Could you check a few things on this model? Use its own coordinates, in mm. Face numbers are marked on the shaded views. A direction names the side the tool comes from. Give positions to 0.01 mm unless a question says otherwise; leave off trailing zeros. Loops run counter-clockwise (first coordinate to the right, second up) from the corner with the lowest first, then second, coordinate; pieces in that order, holes last. Notation, with made-up numbers: (-15.75, 23.5) - (-9.75, 23.5) arc R24 cw to (-9.75, 48.5) - close; hole circle Ø4 at (46, 63). An arc over 180 degrees is marked (long way). Write each question's results on one line, items separated by ' | '. Start each with the question number.
```python
from build123d import *
from build123d.topology import SkipClean

# Parameters (mm, degrees)
SKETCH_1_R          = 1.000029699
SKETCH_1_R_2        = 1.000000092
EXTRUDE_1_DEPTH     = 5
SKETCH_2_W          = 21.526040124
SKETCH_2_H          = 12.5
EXTRUDE_2_DEPTH     = 1.68
SKETCH_3_R          = 0.95
CUT_EXTRUDE_1_DEPTH = 5
SKETCH_4_W          = 12
SKETCH_4_H          = 4.5
SKETCH_4_R          = 1.000000092
EXTRUDE_3_DEPTH     = 7.05
SKETCH_5_R          = 1.149999977
EXTRUDE_4_DEPTH     = 6
CUT_EXTRUDE_START   = -5
SKETCH_6_R          = 0.95
CUT_EXTRUDE_2_DEPTH = 5
SKETCH_7_R          = 1
CUT_EXTRUDE_3_DEPTH = 100
SKETCH_8_R          = 1
CUT_EXTRUDE_4_DEPTH = 3
CUT_EXTRUDE_START_2 = -3
SKETCH_9_R          = 1
CUT_EXTRUDE_5_DEPTH = 3
CUT_EXTRUDE_6_DEPTH = 3.2
CUT_EXTRUDE_7_DEPTH = 3.2


with BuildPart() as part:
    # 草图1 → 凸台-拉伸1 (new body)
    with BuildSketch(Plane.XY):
        Polygon((21.440408464, 11.835070794), (24.640408464, 11.835070794), (24.640408464, 26.596532095), (-17.959592209, 26.596532095), (-23.959592393, 20.596531911), (-23.959592393, 11.805155949), (-20.759591536, 11.805155949), (-20.759591536, -13.834684697), (-9.38563166, -26.403467905), (12.140408464, -26.403467905), (12.140408464, -13.903467905), (21.440408464, -13.903467905), align=None)
        with Locations((-0.265302528, 18.346532095)):
            Circle(SKETCH_1_R, mode=Mode.SUBTRACT)
        with Locations((12.234697472, 18.346532095)):
            Circle(SKETCH_1_R_2, mode=Mode.SUBTRACT)
        with BuildLine():
            ThreePointArc((11.399532521, -9.103467905), (12.234697472, -10.653468153), (13.069862423, -9.103467905))
            Line((13.069862423, -9.103467905), (14.740408464, -9.103467905))
            Line((14.740408464, -9.103467905), (14.740408464, -7.403467905))
            Line((14.740408464, -7.403467905), (18.740408464, -7.403467905))
            Line((18.740408464, -7.403467905), (18.740408464, 16.096532095))
            Line((18.740408464, 16.096532095), (-6.759591536, 16.096532095))
            Line((-6.759591536, 16.096532095), (-6.759591536, -7.403467905))
            Line((-6.759591536, -7.403467905), (-2.759591536, -7.403467905))
            Line((-2.759591536, -7.403467905), (-2.759591536, -9.103467905))
            Line((-2.759591536, -9.103467905), (-1.105259185, -9.103467905))
            ThreePointArc((-1.105259185, -9.103467905), (-0.265302528, -10.657473475), (0.574654129, -9.103467905))
            Line((0.574654129, -9.103467905), (2.240408464, -9.103467905))
            Line((2.240408464, -9.103467905), (2.240408464, -7.403467905))
            Line((2.240408464, -7.403467905), (9.740408464, -7.403467905))
            Line((9.740408464, -7.403467905), (9.740408464, -9.103467905))
            Line((9.740408464, -9.103467905), (11.399532521, -9.103467905))
        make_face(mode=Mode.SUBTRACT)
    extrude(amount=EXTRUDE_1_DEPTH)

    # 草图2 → 凸台-拉伸2 (add)
    with BuildSketch(Plane.XY.offset(5)):
        with Locations((1.377388402, -20.153467905)):
            Rectangle(SKETCH_2_W, SKETCH_2_H)
    extrude(amount=EXTRUDE_2_DEPTH)

    # 草图3 → 切除-拉伸1 (cut)
    with BuildSketch(Plane.XZ.offset(26.403467905)):
        with Locations((-4.122611598, 3.34)):
            Circle(SKETCH_3_R)
        with Locations((6.877388402, 3.34)):
            Circle(SKETCH_3_R)
    extrude(amount=-CUT_EXTRUDE_1_DEPTH, mode=Mode.SUBTRACT)

    # 草图4 → 凸台-拉伸3 (add)
    # profile 1 of 2: a face of its own
    with SkipClean():  # the faces are left unmerged after this step: merging them gives an invalid solid
        with BuildSketch(Plane.XY.offset(5)):
            with BuildLine():
                Line((6.240408464, -7.403467905), (6.240408464, -11.903467905))
                Line((6.240408464, -11.903467905), (18.240408464, -11.903467905))
                Line((18.240408464, -11.903467905), (18.240408464, -7.403467905))
                Line((18.240408464, -7.403467905), (14.740408464, -7.403467905))
                Line((14.740408464, -7.403467905), (14.740408464, -9.103467905))
                Line((14.740408464, -9.103467905), (13.069862423, -9.103467905))
                ThreePointArc((13.069862423, -9.103467905), (12.234697472, -10.653468153), (11.399532521, -9.103467905))
                Line((11.399532521, -9.103467905), (9.740408464, -9.103467905))
                Line((9.740408464, -9.103467905), (9.740408464, -7.403467905))
                Line((9.740408464, -7.403467905), (6.240408464, -7.403467905))
            make_face()
        # profile 2 of 2: a face of its own
        with BuildSketch(Plane.XY.offset(5)):
            with Locations((12.240408464, 18.346532095)):
                Rectangle(SKETCH_4_W, SKETCH_4_H)
            with Locations((12.234697472, 18.346532095)):
                Circle(SKETCH_4_R, mode=Mode.SUBTRACT)
        extrude(amount=EXTRUDE_3_DEPTH)

    # 草图5 → 凸台-拉伸4 (add)
    # profile 1 of 2: a face of its own
    with SkipClean():  # the faces are left unmerged after this step: merging them gives an invalid solid
        with BuildSketch(Plane(origin=(0, 20.596532095, 0), x_dir=(1, 0, 0), z_dir=(0, 1, 0))):
            Polygon((-9.07755609, -5), (-3.077555613, -18.999999523), (-3.077555613, -23.999999285), (5.440409227, -23.999999285), (13.490934884, -12.05), (6.240408464, -12.05), (6.240408464, -5), align=None)
            with Locations(Location((0.328667587, -21.535050638, 0), (0, 0, 270))):
                Circle(SKETCH_5_R, mode=Mode.SUBTRACT)
        # profile 2 of 2: a face of its own
        with BuildSketch(Plane(origin=(0, 20.596532095, 0), x_dir=(1, 0, 0), z_dir=(0, 1, 0))):
            Polygon((18.240408464, -5), (6.240408464, -5), (6.240408464, -12.05), (13.490934884, -12.05), align=None)
        extrude(amount=EXTRUDE_4_DEPTH)

    # 草图6 → 切除-拉伸2 (cut)
    with SkipClean():  # the faces are left unmerged after this step: merging them gives an invalid solid
        with BuildSketch(Plane(origin=(0, 26.596532095, 0), x_dir=(1, 0, 0), z_dir=(0, 1, 0)).offset(CUT_EXTRUDE_START)):
            with Locations((-4.122611598, -3.34)):
                Circle(SKETCH_6_R)
            with Locations((6.877388402, -3.34)):
                Circle(SKETCH_6_R)
        extrude(amount=CUT_EXTRUDE_2_DEPTH, mode=Mode.SUBTRACT)

    # 草图7 → 切除-拉伸3 (cut)
    with SkipClean():  # the faces are left unmerged after this step: merging them gives an invalid solid
        with BuildSketch(Plane(origin=(21.440408464, 0, 0), x_dir=(0, 0, -1), z_dir=(1, 0, 0))):
            with Locations(Location((-2.5, 8.935070794, 0), (0, 0, 90))):
                Circle(SKETCH_7_R)
            with Locations(Location((-2.5, -0.064929206, 0), (0, 0, 90))):
                Circle(SKETCH_7_R)
        extrude(amount=-CUT_EXTRUDE_3_DEPTH, mode=Mode.SUBTRACT)

    # 草图8 → 切除-拉伸4 (cut)
    with SkipClean():  # the faces are left unmerged after this step: merging them gives an invalid solid
        with BuildSketch(Plane(origin=(21.440408464, 0, 0), x_dir=(0, 0, -1), z_dir=(1, 0, 0))):
            with Locations(Location((-2.5, -9.064929206, 0), (0, 0, 90))):
                Circle(SKETCH_8_R)
        extrude(amount=-CUT_EXTRUDE_4_DEPTH, mode=Mode.SUBTRACT)

    # 草图9 → 切除-拉伸5 (cut)
    with SkipClean():  # the faces are left unmerged after this step: merging them gives an invalid solid
        with BuildSketch(Plane.ZY.offset(20.759591536).offset(CUT_EXTRUDE_START_2)):
            with Locations(Location((2.5, -9.064929206, 0), (0, 0, 90))):
                Circle(SKETCH_9_R)
        extrude(amount=CUT_EXTRUDE_5_DEPTH, mode=Mode.SUBTRACT)

    # 草图10 → 切除-拉伸6 (cut)
    with SkipClean():  # the faces are left unmerged after this step: merging them gives an invalid solid
        with BuildSketch(Plane.ZY.offset(23.959592393)):
            Polygon((5, 11.805155949), (0, 11.805155949), (5, 14.691907295), align=None)
        extrude(amount=-CUT_EXTRUDE_6_DEPTH, mode=Mode.SUBTRACT)

    # 草图11 → 切除-拉伸7 (cut)
    with SkipClean():  # the faces are left unmerged after this step: merging them gives an invalid solid
        with BuildSketch(Plane(origin=(24.640408464, 0, 0), x_dir=(0, 0, -1), z_dir=(1, 0, 0))):
            Polygon((0, 11.835070794), (-5, 14.72182214), (-5, 11.835070794), align=None)
        extrude(amount=-CUT_EXTRUDE_7_DEPTH, mode=Mode.SUBTRACT)


solid = part.part
```
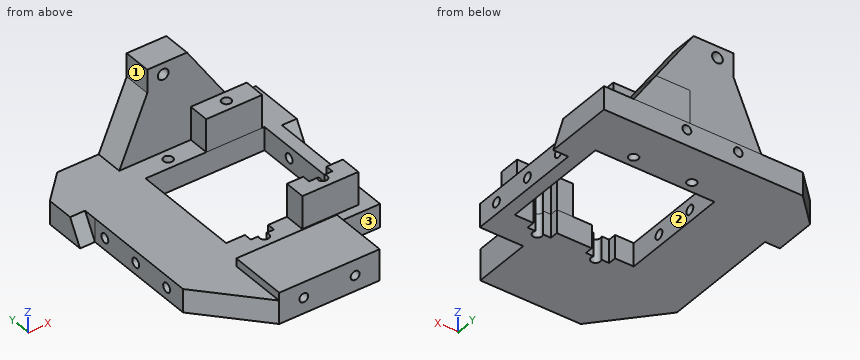
Q1. I want a section at A-A, the plane y = -3.5. List the corners of the cut face in (x, z) for me.
Q2. Which directions (+Z, -Z, +X, -X, +Y, -Y) give clear straight access to the entire face, cutting with the end or side of a thin tool? Please do the marked faces 1, 2 and 3.
Q3. I want a section at B-B, the plane z = 8.5. List the corners of the cut face in (x, y) for me.
Q4. I need wall thicknesses on L1, parallel to Y at x = -5.5, z = 1.25; L2, parallel to X at y = 4.5, z = 3.75; L3, parallel to Z at x = 4.5, y = 19.5. Which ranges of each line are inside material? Lowest first, please. Write a range as from..to.
Q5. I'm going to push flat-ended pins straight in: pin 1 Ø2 at (x, y) = (-10, -13.5) entering from +Z; pin 2 Ø2.5 at (x, y) = (12.23, 18.35) entering from +Z; pin 3 Ø1.3 at (y, z) = (-9, 9) entering from -X. Where does each tip first touch, or does it pass through?
Q6. I want a section at C-C, the plane x = -14.5. List the corners of the cut face in (y, z) for me.
Q7. I want a section at D-D, the plane z = 13.75. List the corners of the cut face in (x, y) for me, then the cut area to 3 significant figures.
Conclusion:
1) outline: (-20.76, 0) - (-6.76, 0) - (-6.76, 5) - (-20.76, 5) - close; (18.74, 0) - (21.44, 0) - (21.44, 5) - (18.74, 5) - close
2) face 1: +Z, -X, +Y, -Y | face 2: +Z, -Z | face 3: +Z, -Z, +X, -Y
3) outline: (-7.58, 20.6) - (6.24, 20.6) - (6.24, 16.1) - (18.24, 16.1) - (18.24, 20.6) - (15.88, 20.6) - (15.88, 26.6) - (-7.58, 26.6) - close; (6.24, -11.9) - (18.24, -11.9) - (18.24, -7.4) - (14.74, -7.4) - (14.74, -9.1) - (13.07, -9.1) arc R1 cw (long way) to (11.4, -9.1) - (9.74, -9.1) - (9.74, -7.4) - (6.24, -7.4) - close; hole circle Ø2 at (12.23, 18.35)
4) L1: -26.4..-7.4, 16.1..26.6 | L2: -20.76..-6.76, 18.74..21.44 | L3: 0..5
5) pin 1: z = 6.68 | pin 2: z = 12.05 | pin 3: x = 6.24
6) outline: (-20.75, 0) - (26.6, 0) - (26.6, 5) - (-20.75, 5) - close; hole circle Ø2 at (-0.06, 2.5); hole circle Ø2 at (8.94, 2.5)
7) outline: (-5.33, 20.6) - (12.35, 20.6) - (12.35, 26.6) - (-5.33, 26.6) - close | area: 106 mm^2
